CAD build for the part. Positions are in the model's coordinates, mm. Round coordinates to 2 decimals unless told otherwise and drop trailing zeros. Order: outer loops, then holes, each group sorted by start corner. A loop starts at its lowest first (then second) coordinate and runs counter-clockwise, first axis right, second up. Notation, with made-up numbers: (31.25, 59) -> (67.25, 59) arc R23 cw to (67.25, 76) -> close; hole circle Ø2 at (-19.5, 49). An arc over 180 degrees is marked (long way). Answer as CSV lines item,"result". Start each with the question number.
Autodesk Inventor part; units mm, degrees
ref_plane "Arbeitsebene1" through (0, 3, 0) normal (0, -1, 0) x (1, 0, 0)
ref_plane "Arbeitsebene2" through (0, 0.25, 0) normal (0, -1, 0) x (1, 0, 0)
ref_plane "YZ Plane" through (0, 0, 0) normal (1, 0, 0) x (0, 1, 0)
sketch "Skizze2" plane through (0, 0, 0) normal (0, 1, 0) x (-1, 0, 0)
  line L0 (0, 0) -> (-0.6, 0)
  line L1 (-0.6, 0) -> (-0.6, 0.6)
  line L2 (-0.6, 0.6) -> (0, 0.6)
  line L3 (0, 0.6) -> (0, 0)
  dimension "d0" = 0.6
  dimension "d1" = 0.6
extrude "Extrusion1" add sketch "Skizze2" along normal blind 11
ref_plane "Arbeitsebene1" through (0, 3, 0) normal (0, -1, 0) x (1, 0, 0)
sketch "Skizze3" plane through (0, 3, 0) normal (0, -1, 0) x (1, 0, 0)
  line L0 (1.57, 1.57) -> (-0.97, 1.57)
  line L1 (-0.97, 1.57) -> (-0.97, -0.97)
  line L2 (-0.97, -0.97) -> (1.57, -0.97)
  line L3 (1.57, -0.97) -> (1.57, 1.57)
  line L4 (0.6, 0) -> (0.6, 0.6)
  line L5 (0, 0.6) -> (0.6, 0.6)
  point P0 (0, 0)
  dimension "d5" = 2.54
  dimension "d6" = 2.54
  dimension "d7" = 0.97
  dimension "d8" = 0.97
extrude "Extrusion2" add sketch "Skizze3" against normal blind 2.5
chamfer "Fase1" distance 0.25 angle 45 4 edges at (-0.97, 4.25, -0.97) (1.57, 4.25, -0.97) (1.57, 4.25, 1.57) (-0.97, 4.25, 1.57)
chamfer "Fase2" distance 0.15 angle 45 4 edges at (0.6, 0, 0.3) (0.3, 0, 0) (0, 0, 0.3) (0.3, 0, 0.6)
chamfer "Fase3" distance 0.15 angle 45 4 edges at (0.6, 11, 0.3) (0.3, 11, 0) (0, 11, 0.3) (0.3, 11, 0.6)
ref_plane "Arbeitsebene2" through (0, 0.25, 0) normal (0, -1, 0) x (1, 0, 0)
sketch "Skizze6" plane through (0, 0.25, 0) normal (0, -1, 0) x (1, 0, 0)
  circle A0 centre (0.3, 0.3) radius 0.325
  line L0 (0, 0) -> (0.6, 0)
  line L1 (0.6, 0) -> (0.6, 0.6)
  dimension "d26" = 0.65
  dimension "d27" = 0.3
  dimension "d28" = 0.3
extrude "Extrusion4" add sketch "Skizze6" against normal blind 0.5 contours A0 L1 | L1 A0 L0 | L0 A0 picked at (0.4269, 0.2422)
properties part number "Pin"
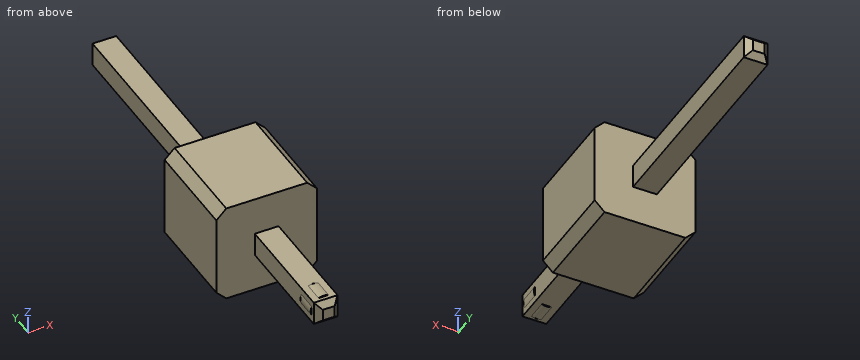
Item 1: Band-saw the part on C-C, the plane x = -0.3. Give the cut face in (y, z).
Item 2: Pin check, flat tips, straight feed: pin 1 (0.5 mm diameter, centred on x = 0.5, y = 7, fed in from -Z); pin 2 (1 mm diameter, centred on x = 1, z = 0.5, fed in from -Y); pin 3 (0.7 mm diameter, centred on x = 0, y = 9, fed in from +Z). Stop position of each tip, or through.
Item 3: Band-saw the part on A-A, the plane y = 4.5. Give the cut face in (x, z).
Item 4: Band-saw the part on B-B, the plane z = -0.2. Give the cut face in (x, y).
Item 5: Probe line 1 (Y direction, x = 1.15, z = 0.55); line 2 (Z direction, x = 0.05, y = 6.75). List the from-to ranges inside material, lowest first.
Values:
1,outline,"(3, -0.97) -> (5.5, -0.97) -> (5.5, 1.57) -> (3, 1.57) -> close"
2,pin 1,"z = 0"
2,pin 2,"y = 0.05"
2,pin 3,"z = 0.6"
3,outline,"(-0.97, -0.72) -> (-0.72, -0.97) -> (1.32, -0.97) -> (1.57, -0.72) -> (1.57, 1.32) -> (1.32, 1.57) -> (-0.72, 1.57) -> (-0.97, 1.32) -> close"
4,outline,"(-0.97, 3) -> (1.57, 3) -> (1.57, 5.5) -> (-0.97, 5.5) -> close"
5,line 1,"3 to 5.5"
5,line 2,"0 to 0.6"
